from build123d import *

# Parameters (mm, degrees)
SKETCH1_R           = 47
SKETCH1_R_2         = 43
BOSS_EXTRUDE1_DEPTH = 1.5
CUT_EXTRUDE1_DEPTH  = 100


with BuildPart() as part:
    # Sketch1 → Boss-Extrude1 (new, symmetric)
    with BuildSketch(Plane(origin=(0, 0, 0), x_dir=(0, 1, 0), z_dir=(0, 0, 1))):
        with Locations(Location((0, 0, 0), (0, 0, 270))):
            Circle(SKETCH1_R)
        with Locations(Location((0, 0, 0), (0, 0, 270))):
            Circle(SKETCH1_R_2, mode=Mode.SUBTRACT)
    extrude(amount=BOSS_EXTRUDE1_DEPTH, both=True)

    # Sketch4 → Cut-Extrude1 (cut)
    with BuildSketch(Plane(origin=(0, 0, 0), x_dir=(-1, 0, 0), z_dir=(0, 1, 0))):
        Polygon((19.908984976, 1.5), (22.908984976, -1.5), (24.323198539, -1.5), (21.323198539, 1.5), align=None)
    extrude(amount=CUT_EXTRUDE1_DEPTH, mode=Mode.SUBTRACT)


solid = part.part
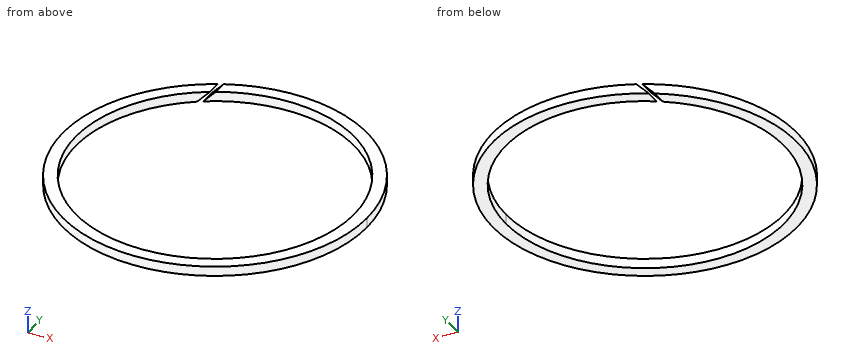
Work out the finished part from the listing and answer in its coordinate system (mm). Give positions to 0.01 mm unless a question says otherwise; leave off trailing zeros. Order: outer loops, then holes, each group sorted by start corner. A loop starts at its lowest first (then second) coordinate and runs counter-clockwise, first axis right, second up. Notation, with made-up numbers: (80.25, 76.5) - (115.25, 76.5) arc R30 ccw to (115.25, 100.5) - close; hole circle Ø1 at (-4, 9.5). An arc over 180 degrees is marked (long way). Answer as CSV lines item,"result". Start each with the question number.
Q1. The part is cut by section A-A (x = -26.5). Write down the section's boundary in (y, z), then the cut area to 3 significant figures.
Q2. Given pin 1 Ø8 at (x, y) = (24, -35.5) entering from +Z; pin 2 Ø1 at (x, z) = (-4, 0.5) entering from +Y; pin 3 Ø1.5 at (x, z) = (4, 0) entering from -Y, each flat-ended and moving along its own axis, determine where each tip first touches the part or whether it passes through.
Q3. The part is cut by section B-B (y = 14). Write down the section's boundary in (x, z).
Q4. Find the intervals of material crossed by L1, parallel to Y at x = 0, z = 0.85; L2, parallel to Y at x = 28.5, z = 1.15; L3, parallel to X at y = 10, z = -0.9, in increasing order. Write a range as [from, to].
Q5. The part is cut by section C-C (z = -0.7). Write down the section's boundary in (x, y).
Check result:
1,outline,"(-38.82, -1.5) - (-33.86, -1.5) - (-33.86, 1.5) - (-38.82, 1.5) - close; (33.86, -1.5) - (38.82, -1.5) - (38.82, 1.5) - (33.86, 1.5) - close"
1,area,"29.7 mm²"
2,pin 1,"stops at z = 1.5"
2,pin 2,"stops at y = 46.87"
2,pin 3,"stops at y = -46.89"
3,outline,"(-44.87, -1.5) - (-40.66, -1.5) - (-40.66, 1.5) - (-44.87, 1.5) - close; (40.66, -1.5) - (44.87, -1.5) - (44.87, 1.5) - (40.66, 1.5) - close"
4,L1,"y = [-47, -43], [43, 47]"
4,L2,"y = [-37.37, -32.2], [32.2, 37.37]"
4,L3,"x = [-45.92, -41.82], [41.82, 45.92]"
5,outline,"(-23.52, 36) - (-23.52, 40.69) arc R47 ccw (long way) to (-22.11, 41.48) - (-22.11, 36.88) arc R43 cw (long way) to start"
